Part model, mm, in its own coordinate system. Face numbers are marked on the shaded views. A direction names the side the tool comes from. Coordinates: 2 decimals unless noted, no trailing zeros. Order: outer loops, then holes, each group sorted by start corner. A loop starts at its lowest first (then second) coordinate and runs counter-clockwise, first axis right, second up. Notation, with made-up numbers: M 43,70.25 L 98,70.25 A30 ccw 98,104.25 Z; hole C 65.5,-3 d8. An arc over 180 degrees is marked long. Answer in a Markdown table with one row per item. Add a question column.
from build123d import *

# Parameters (mm, degrees)
SKETCH_2_W      = 46
SKETCH_2_H      = 21.5
EXTRUDE_1_DEPTH = 32
SKETCH_3_R      = 5
EXTRUDE_2_DEPTH = 2
SKETCH_4_R      = 3
EXTRUDE_3_DEPTH = 14
SKETCH_5_R      = 12
EXTRUDE_4_DEPTH = 30.8


with BuildPart() as part:
    # 草图2 → 凸台-拉伸1 (new body)
    with BuildSketch(Plane.XY):
        with Locations((2.647117171, 17.006037157)):
            Rectangle(SKETCH_2_W, SKETCH_2_H)
    extrude(amount=EXTRUDE_1_DEPTH)

    # 草图3 → 凸台-拉伸2 (add)
    with BuildSketch(Plane(origin=(0, 27.756037157, 0), x_dir=(1, 0, 0), z_dir=(0, 1, 0))):
        with Locations((-7.352882829, -16)):
            Circle(SKETCH_3_R)
    extrude_2 = extrude(amount=EXTRUDE_2_DEPTH)

    # 草图4 → 凸台-拉伸3 (add)
    with BuildSketch(Plane(origin=(0, 29.756037157, 0), x_dir=(1, 0, 0), z_dir=(0, 1, 0))):
        with Locations((-7.352882829, -16)):
            Circle(SKETCH_4_R)
    extrude_3 = extrude(amount=EXTRUDE_3_DEPTH)

    # 镜向1: 凸台-拉伸2, 凸台-拉伸3 across plane
    add(extrude_2.mirror(Plane.ZX.offset(17.506037157)))
    add(extrude_3.mirror(Plane.ZX.offset(17.506037157)))

    # 草图5 → 凸台-拉伸4 (add)
    with BuildSketch(Plane(origin=(25.647117171, 0, 0), x_dir=(0, 0, -1), z_dir=(1, 0, 0))):
        with Locations((-16, 17.506037157)):
            Circle(SKETCH_5_R)
    extrude(amount=EXTRUDE_4_DEPTH)


solid = part.part
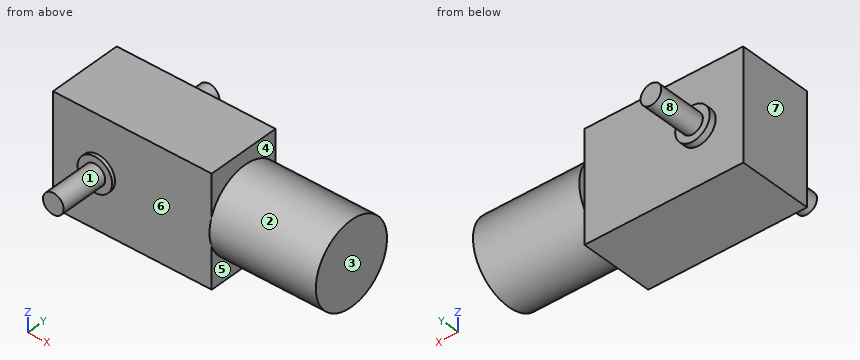
(1) Wall check: line 1 (X direction, y = 15.5, z = 29); line 2 (Y direction, x = 7, z = 12.5); line 3 (X direction, y = 5.5, z = 20). Give the ranges that are in metal, low to high.
(2) Pull direction X, two halves, no side cores. Call the marked faces 6, 7 and 8: pulls with the +X half, pulls with the -X half, needs draft (parallel to the pull), parting line crosses it, or undercut.
(3) Slice it at C-C (x = -14). List the corners of the cut face in (y, z).
(4) Slice it at B-B (y = 12.5). List the corners of the cut face in (x, z), and give its area (3 significant figures).
(5) 3-axis set-ups, long thin cutter, end or side, ignore diameter. For the marked faces 1, 2, 3, 4 and 5: which of +Z, -Z, +X, -X, +Y, -Y reach the whole face in a straight line?
(6) Drop flat-ended pins along their axis: P1, Ø1.5, axis at x = 41.5, z = 16.5, coming from the +Y side; P2, Ø0.9, axis at y = 28.5, z = 16, coming from the -X side; P3, Ø8, axis at x = 21.5, z = 25.5, coming from the +Y side. Give the stop position or say it passes through.
(7) Slice it at A-A (z = 16). List the corners of the cut face in (x, y), and give its area (3 significant figures).
(8) Slice it at D-D (z = 26.5). List the corners of the cut face in (x, y).
Computed:
| question | item | result |
|---|---|---|
| 1 | line 1 | x = -20.35 to 25.65 |
| 1 | line 2 | y = 6.26 to 27.76 |
| 1 | line 3 | x = -10.35 to -4.35 |
| 2 | face 6 | undercut |
| 2 | face 7 | pulls with the -X half |
| 2 | face 8 | parting line crosses it |
| 3 | outline | M 6.26,0 L 27.76,0 L 27.76,32 L 6.26,32 Z |
| 4 | outline | M -20.35,0 L 25.65,0 L 25.65,5.09 L 56.45,5.09 L 56.45,26.91 L 25.65,26.91 L 25.65,32 L -20.35,32 Z |
| 4 | area | 2,140 mm^2 |
| 5 | face 1 | -Y |
| 5 | face 2 | +X |
| 5 | face 3 | +Z, -Z, +X, +Y, -Y |
| 5 | face 4 | +Z, +X |
| 5 | face 5 | -Z, +X |
| 6 | P1 | stops at y = 29.51 |
| 6 | P2 | stops at x = -12.35 |
| 6 | P3 | stops at y = 27.76 |
| 7 | outline | M -20.35,6.26 L -12.35,6.26 L -12.35,5.26 L -10.35,5.26 L -10.35,-8.74 L -4.35,-8.74 L -4.35,5.26 L -2.35,5.26 L -2.35,6.26 L 25.65,6.26 L 25.65,5.51 L 56.45,5.51 L 56.45,29.51 L 25.65,29.51 L 25.65,27.76 L -2.35,27.76 L -2.35,29.76 L -4.35,29.76 L -4.35,43.76 L -10.35,43.76 L -10.35,29.76 L -12.35,29.76 L -12.35,27.76 L -20.35,27.76 Z |
| 7 | area | 1,930 mm^2 |
| 8 | outline | M -20.35,6.26 L 25.65,6.26 L 25.65,11.7 L 56.45,11.7 L 56.45,23.32 L 25.65,23.32 L 25.65,27.76 L -20.35,27.76 Z |
